from build123d import *

# Parameters (mm, degrees)
SKETCH1_R           = 1.45
BOSS_EXTRUDE2_DEPTH = 2.9


with BuildPart() as part:
    # Sketch1 → Boss-Extrude2 (new body)
    with BuildSketch(Plane.XY):
        Polygon((-53.5, -47.5), (-45.8, -47.5), (-45.8, -67.5), (45.8, -67.5), (45.8, -47.5), (53.5, -47.5), (53.5, 47.5), (45.803905178, 47.5), (45.803905178, 62.5), (-45.8, 62.5), (-45.8, 47.5), (-53.5, 47.5), align=None)
        with Locations((35, -57.5)):
            Circle(SKETCH1_R, mode=Mode.SUBTRACT)
        with Locations((35, 28.5)):
            Circle(SKETCH1_R, mode=Mode.SUBTRACT)
        with Locations((-23, -57.5)):
            Circle(SKETCH1_R, mode=Mode.SUBTRACT)
        with Locations((-23, 28.5)):
            Circle(SKETCH1_R, mode=Mode.SUBTRACT)
        with BuildLine():
            Line((-27.063854383, 61.5), (27.063854383, 61.5))
            ThreePointArc((27.063854383, 61.5), (28.063854383, 60.5), (27.063854383, 59.5))
            Line((27.063854383, 59.5), (-27.063854383, 59.5))
            ThreePointArc((-27.063854383, 59.5), (-28.063854383, 60.5), (-27.063854383, 61.5))
        make_face(mode=Mode.SUBTRACT)
        with BuildLine():
            Line((-27.063854383, 41.5), (27.063854383, 41.5))
            ThreePointArc((27.063854383, 41.5), (28.063854383, 42.5), (27.063854383, 43.5))
            Line((27.063854383, 43.5), (-27.063854383, 43.5))
            ThreePointArc((-27.063854383, 43.5), (-28.063854383, 42.5), (-27.063854383, 41.5))
        make_face(mode=Mode.SUBTRACT)
        with BuildLine():
            Line((-41.456619421, 55.059017376), (-41.456619421, 47.940982624))
            ThreePointArc((-41.456619421, 47.940982624), (-42.456619421, 46.940982624), (-43.456619421, 47.940982624))
            Line((-43.456619421, 47.940982624), (-43.456619421, 55.059017376))
            ThreePointArc((-43.456619421, 55.059017376), (-42.456619421, 56.059017376), (-41.456619421, 55.059017376))
        make_face(mode=Mode.SUBTRACT)
        with BuildLine():
            Line((41.456619421, 55.059017376), (41.456619421, 47.940982624))
            ThreePointArc((41.456619421, 47.940982624), (42.456619421, 46.940982624), (43.456619421, 47.940982624))
            Line((43.456619421, 47.940982624), (43.456619421, 55.059017376))
            ThreePointArc((43.456619421, 55.059017376), (42.456619421, 56.059017376), (41.456619421, 55.059017376))
        make_face(mode=Mode.SUBTRACT)
    extrude(amount=BOSS_EXTRUDE2_DEPTH)


solid = part.part
Geometry: final body of the model. Coordinates: model frame, mm. A direction names the side the tool comes from. Round coordinates to 2 decimals unless told otherwise and drop trailing zeros. Order: outer loops, then holes, each group sorted by start corner. A loop starts at its lowest first (then second) coordinate and runs counter-clockwise, first axis right, second up. Notation, with made-up numbers: (87.25, 32.25) -> (109.25, 32.25) arc R12 ccw to (109.25, 49.25) -> close; hole circle Ø9 at (32, -4.5). An arc over 180 degrees is marked (long way). Put each result on its own line as item: value. Start each with the question number.
Q1. Section B-B on z = 0.9. Give the number of separate pieces and of enclosed holes in the cut face, and give its area (3 significant figures).
Q2. Section A-A on y = -57.5. Return the cut outline in (x, z), and give its area (3 significant figures).
Q3. First-contact query: pin 1 (0.9 mm diameter, centred on x = 49.5, z = 1.5, fed in from +Y); pin 2 (0.9 mm diameter, centred on x = 51, z = 1, fed in from -Y); pin 3 (1.4 mm diameter, centred on y = -58.5, z = 1.5, fed in from +X). Flat tips, straight axial feed; report the tip coordinate or a pass-through.
Q4. Reachability of faces 1 (the flat face through (-45.8, 55, 1)), 2 (the flat face through (45.8, -58, 1)), 3 (the flat face through (0, 59.5, 1)), 4 (the flat face through (-50, -47.5, 1)) from +Z, -Z, +X, -X, +Y, -Y: full face, straight path, thin tool, end or side. Return the list, or none.
Q5. Pull-direction query (X, two-part tool) for faces 5 (the flat face through (50, -47.5, 1)), 6 (the flat face through (-45.8, -57, 1)), 7 (the cylindrical face through (-22.331, 27.214, 1.43)); classes: +X half, -X half, draft (parallel to the pull), parting line (faces both ways), or undercut.
Q6. Line query: probe 1 along Y at (x, z) = (25.5, 2.4); probe 2 along Y at (x, z) = (-23, 1); probe 3 along Y at (x, z) = (35, 2.2). Output: solid intervals per line, ascending.
Q7. Section C-C on x = 35. Return the cut outline in (y, z).
Ans:
1. separate pieces: 1
1. enclosed holes: 8
1. area: 13,100 mm2
2. outline: (-45.8, 0) -> (-24.45, 0) -> (-24.45, 2.9) -> (-45.8, 2.9) -> close; (-21.55, 0) -> (33.55, 0) -> (33.55, 2.9) -> (-21.55, 2.9) -> close; (36.45, 0) -> (45.8, 0) -> (45.8, 2.9) -> (36.45, 2.9) -> close
2. area: 249 mm2
3. pin 1: stops at y = 47.5
3. pin 2: stops at y = -47.5
3. pin 3: stops at x = 45.8
4. face 1: +Z, -Z, -X, +Y
4. face 2: +Z, -Z, +X, -Y
4. face 3: +Z, -Z
4. face 4: +Z, -Z, -X, -Y
5. face 5: draft
5. face 6: -X half
5. face 7: undercut
6. probe 1: y = -67.5 to 41.5, 43.5 to 59.5, 61.5 to 62.5
6. probe 2: y = -67.5 to -58.95, -56.05 to 27.05, 29.95 to 41.5, 43.5 to 59.5, 61.5 to 62.5
6. probe 3: y = -67.5 to -58.95, -56.05 to 27.05, 29.95 to 62.5
7. outline: (-67.5, 0) -> (-58.95, 0) -> (-58.95, 2.9) -> (-67.5, 2.9) -> close; (-56.05, 0) -> (27.05, 0) -> (27.05, 2.9) -> (-56.05, 2.9) -> close; (29.95, 0) -> (62.5, 0) -> (62.5, 2.9) -> (29.95, 2.9) -> close
